Autodesk Inventor part; units mm, degrees
ref_plane "YZ Plane" through (0, 0, 0) normal (1, 0, 0) x (0, 1, 0)
ref_plane "XZ Plane" through (0, 0, 0) normal (0, 1, 0) x (-1, 0, 0)
ref_plane "XY Plane" through (0, 0, 0) normal (0, 0, 1) x (1, 0, 0)
sketch "Sketch1" plane through (0, 0, 0) normal (0, 1, 0) x (-1, 0, 0)
  point P0 (0, 0)
sketch "Sketch2" plane through (0, 0, 0) normal (0, 1, 0) x (-1, 0, 0)
  line L0 (3.3, 8) -> (-3.3, 8)
  line L1 (-3.3, 8) -> (-3.3, -8)
  line L2 (-3.3, -8) -> (3.3, -8)
  line L3 (3.3, -8) -> (3.3, 8)
  line L4 (3.3, 8) -> (-3.3, -8) construction
  line L5 (-3.3, 8) -> (3.3, -8) construction
  point P0 (0, 0)
  dimension "d0" = 6.6
  dimension "d1" = 16
extrude "Extrusion1" add sketch "Sketch2" along normal blind 6.35
sketch "Sketch3" plane through (0, 0, 0) normal (0, -1, 0) x (1, 0, 0)
  line L0 (-8, -8) -> (8, -8)
  line L1 (8, -8) -> (8, 8)
  line L2 (8, 8) -> (-8, 8)
  line L3 (-8, 8) -> (-8, -8)
  line L4 (-8, -8) -> (8, 8) construction
  line L5 (8, -8) -> (-8, 8) construction
  point P0 (0, 0)
  dimension "d13" = 16
  dimension "d14" = 16
move or copy body "Move1" bodies to move or copy 1 copy no translate (0, 6.35, 0)
extrude "Extrusion2" add sketch "Sketch3" against normal up to surface (6.35 mm away)
chamfer "Chamfer1" [suppressed]
chamfer "Chamfer2" [suppressed]
sketch "Sketch4" plane through (-3.3, 12.7, -8) normal (0, 1, 0) x (1, 0, 0)
  line L0 (4.4354, -16) -> (2.1646, -16)
  line L1 (-4.7, 0) -> (11.3, 0)
  point P0 (3.3, -8)
  point P1 (3.3, -3.175)
  point P2 (3.3, -12.825)
fillet "Fillet1" [suppressed]
sketch "Sketch5" plane through (-3.3, 12.7, 8) normal (0, 0, 1) x (1, 0, 0)
  circle A0 centre (3.3, -9.5232) radius 2.9337
  point P0 (3.3, -12.7)
extrude "Extrusion3" [suppressed]
hole "Hole3" [suppressed]
chamfer "Chamfer3" [suppressed]
sketch "Sketch6" plane through (-3.3, 12.7, -8) normal (-1, 0, 0) x (0, 0, 1)
  line L0 (0, 0) -> (16, 0)
  circle A0 centre (8, -2.27) radius 1.27
  point P0 (8, -12.7)
  dimension "d62" = 2.54
extrude "Extrusion4" cut sketch "Sketch6" against normal blind 3.3
sketch "Sketch7" plane through (-3.3, 12.7, 8) normal (0, 0, 1) x (1, 0, 0)
  line L0 (0, -6.35) -> (0, 0)
  line L1 (11.3, -12.7) -> (-4.7, -12.7)
  line L2 (0, -6.35) -> (6.6, -6.35)
  line L3 (6.6, -6.35) -> (6.6, -12.7)
  line L4 (6.6, -12.7) -> (0, -12.7)
  line L5 (0, -12.7) -> (0, -6.35)
  point P0 (3.3, -12.7)
  dimension "d65" = 6.6
extrude "Extrusion5" add sketch "Sketch7" along normal blind 6.35
sketch "Sketch8" plane through (0, 0, 0) normal (0, -1, 0) x (1, 0, 0)
  line L0 (-8, 8) -> (-8, -8)
  line L1 (-8, -8) -> (-8, 8)
  line L2 (-3.3, 8) -> (-8, 8)
  line L3 (-8, 8) -> (-3.3, 8)
  line L4 (-3.3, 8) -> (-3.3, 14.35)
  line L5 (-3.3, 8) -> (-3.3, 14.35)
  line L6 (3.3, 14.35) -> (-3.3, 14.35)
  line L7 (-3.3, 14.35) -> (3.3, 14.35)
  line L8 (8, 8) -> (3.3, 8)
  line L9 (3.3, 14.35) -> (3.3, 8)
  line L10 (3.3, 8) -> (8, 8)
  line L11 (-8, -8) -> (8, -8)
  line L12 (8, 8) -> (8, -8)
  line L13 (8, -8) -> (-8, -8)
  point P0 (0, 0)
hole "Hole4" at (0, 12.7, 4.825) at (0, 12.7, -4.825) direction (0, -1, 0) diameter 2.946 end through all
extrude "Extrusion6" cut sketch "Sketch8" against normal blind 1.35
hole "Hole6" at (0, 3.85, 14.35) direction (0, 0, -1) diameter 2.1565 depth 6.35
sketch "Sketch9" plane through (0, 1.35, 0) normal (0, -1, 0) x (1, 0, 0)
  point P0 (0, 0)
  point P1 (0, 0)
properties part number "copper_top_ledgereod" material "Copper"
Geometry: final body of the model. Coordinates: model frame, mm. A direction names the side the tool comes from. Round coordinates to 2 decimals unless told otherwise and drop trailing zeros. Write each loop counter-clockwise with the first axis right and the second up, starting at its lowest first coordinate (ties: lowest second). Pieces come first, ordered by that corner, then holes. Notation, with made-up numbers: M 52,-1.75 L 100,-1.75 A30 ccw 100,35.25 Z; hole C 69.25,70 d11. An arc over 180 degrees is marked long. Answer in a Markdown table with one row per item. Add a question column.
(1) Cut plane D-D, the plane y = 10.43. Return the cut outline in (x, z) (3 decimals).
(2) Contact query for flat-ended pins moving along their axis: pin 1 (3 mm diameter, centred on y = 10.5, z = 1.5, fed in from +X); pin 2 (2.5 mm diameter, centred on y = 3.5, z = 10.5, fed in from -X); pin 3 (1.8 mm diameter, centred on x = 0, z = 4.825, fed in from +Y); pin 4 (4 mm diameter, centred on x = -6, y = 5, fed in from +Z). Output: stop coordinate, or through.
(3) Cut plane C-C, the plane z = 0. Return the cut outline in (x, y).
(4) Reachability of faces 1 (the face through (3.3, 4, 11)), 2 (the face through (3.3, 9, 0)), 3 (the face through (0, 6.35, 11)), 4 (the face through (-3.3, 4, 11)) from +Z, -Z, +X, -X, +Y, -Y: full face, straight path, thin tool, end or side. Return the list, or none.
(5) Cut plane A-A, the plane y = 3.85. Return the cut outline in (x, z) (3 decimals).
(6) Ray query, L1, parallel to Z at x = 0, y = 7.5; L2, parallel to X at y = 3.85, z = 13; L3, parallel to Z at x = 0.5, y = 10.75. Return the intervals inside material, ascending.
(7) Cut plane B-B, the plane z = 9.5. Return the cut outline in (x, y).
(8) Draft query along Z for faces 5 (the face through (1, 5, 14.35)), 6 (the face through (0, 6, -8)), 7 (the face through (0, 10, 0)). Return one class per face: pulls with the +Z half, pulls with the -Z half, needs draft (parallel to the pull), parting line crosses it, or undercut.
Established:
| question | item | result |
|---|---|---|
| 1 | outline | M -3.3,-8 L 3.3,-8 L 3.3,8 L -3.3,8 L -3.3,1.27 L 0,1.27 L 0,-1.27 L -3.3,-1.27 Z; hole C 0,-4.825 d2.946; hole C 0,4.825 d2.946 |
| 2 | pin 1 | x = 3.3 |
| 2 | pin 2 | x = -3.3 |
| 2 | pin 3 | through |
| 2 | pin 4 | z = 8 |
| 3 | outline | M -8,1.35 L 8,1.35 L 8,6.35 L 3.3,6.35 L 3.3,12.7 L -3.3,12.7 L -3.3,11.7 L 0,11.7 L 0,9.16 L -3.3,9.16 L -3.3,6.35 L -8,6.35 Z |
| 4 | face 1 | +Z, +X, +Y, -Y |
| 4 | face 2 | +Z, -Z, +X, +Y |
| 4 | face 3 | +Z, +X, -X, +Y |
| 4 | face 4 | +Z, -X, +Y, -Y |
| 5 | outline | M -8,-8 L 8,-8 L 8,8 L 3.3,8 L 3.3,14.35 L 1.078,14.35 L 1.078,8 L -1.078,8 L -1.078,14.35 L -3.3,14.35 L -3.3,8 L -8,8 Z; hole C 0,-4.825 d2.946; hole C 0,4.825 d2.946 |
| 6 | L1 | -8 to -6.3, -3.35 to 3.35, 6.3 to 8 |
| 6 | L2 | -3.3 to -1.08, 1.08 to 3.3 |
| 6 | L3 | -8 to -6.21, -3.44 to 3.44, 6.21 to 8 |
| 7 | outline | M -3.3,1.35 L 3.3,1.35 L 3.3,6.35 L -3.3,6.35 Z; hole C 0,3.85 d2.16 |
| 8 | face 5 | pulls with the +Z half |
| 8 | face 6 | pulls with the -Z half |
| 8 | face 7 | undercut |
